Can you work these out from the model? Positions are in its coordinate system, mm. A direction names the side the tool comes from. Give positions to 0.01 mm unless a question says otherwise; leave off trailing zeros. Order: outer loops, then holes, each group sorted by start corner. A loop starts at its lowest first (then second) coordinate and runs counter-clockwise, first axis right, second up. Notation, with made-up numbers: M 21.25,68 L 58.25,68 A26 cw 58.25,98 Z; hole C 22.25,42.25 d7. An arc over 180 degrees is marked long. Answer as a JSON object with one key per item and string values.
```python
from build123d import *

# Parameters (mm, degrees)
F0_W     = 63.144043088
F0_H     = 24.9639227986
F1_DEPTH = 25.4
F2_W     = 1.27
F2_H     = 10.16
F3_DEPTH = 3.175
F4_W     = 10.16
F4_H     = 1.27
F5_DEPTH = 3.175


# Not quite as in the source:
# - a feature names something its author has since deleted; it is built from what else it names


with BuildPart() as f1:
    # F0 (on Front) → F1 (new body, symmetric)
    with BuildSketch(Plane.XZ):
        Rectangle(F0_W, F0_H)
    extrude(amount=F1_DEPTH, both=True)

    # F2 (on Front) → F3 (join, symmetric)
    with BuildSketch(Plane.XZ):
        with Locations((29.0800049829, 17.5400783525)):
            Rectangle(F2_W, F2_H)
    extrude(amount=F3_DEPTH, both=True)

    # F4 (on Front) → F5 (join, symmetric)
    with BuildSketch(Plane.XZ):
        with Locations((-36.6476550698, -9.8343824477)):
            Rectangle(F4_W, F4_H)
    extrude(amount=F5_DEPTH, both=True)


solid = f1.part
```
1) I want a section at A-A on y = -1. Write out the boundary of the cut face in (x, z) (3 decimals), and give its area (3 significant figures).
Results found:
{"outline": "M -41.728,-10.469 L -31.572,-10.469 L -31.572,-12.482 L 31.572,-12.482 L 31.572,12.482 L 29.715,12.482 L 29.715,22.62 L 28.445,22.62 L 28.445,12.482 L -31.572,12.482 L -31.572,-9.199 L -41.728,-9.199 Z", "area": "1,600 mm²"}
2) For faces 1 (the face through (-37, 0, -10.469)), 2 (the face through (29.715, 0, 17)), 3 (the face through (0, 0, -12.482)), 4 (the face through (-37, 0, -9.199)), which set-ups out of +Z, -Z, +X, -X, +Y, -Y let a thin tool reach every point of the face, with its end or its side?
Results found:
{"face 1": "-Z, -X, +Y, -Y", "face 2": "+Z, +X, +Y, -Y", "face 3": "-Z, +X, -X, +Y, -Y", "face 4": "+Z, -X, +Y, -Y"}
3) I'm going to push flat-ended pins straight in: pin 1 Ø1 at (x, z) = (-37.5, -10) entering from +Y (3 decimals); pin 2 Ø0.6 at (x, z) = (29, 16) entering from -Y (3 decimals); pin 3 Ø6 at (x, y) = (-29, -11) entering from +Z. Where does each tip first touch, or does it pass through?
Results found:
{"pin 1": "stops at y = 3.175", "pin 2": "stops at y = -3.175", "pin 3": "stops at z = 12.48"}
4) I need wall thicknesses on L1, parallel to Z at x = 19.5, y = 4.5; L2, parallel to X at y = 1.5, z = 11; L3, parallel to X at y = 0, z = 16 (3 decimals). Which ranges of each line are inside material? Lowest first, please.
Results found:
{"L1": "z = -12.48 to 12.48", "L2": "x = -31.57 to 31.57", "L3": "x = 28.445 to 29.715"}
5) I want a section at B-B on z = 20. Write out the boundary of the cut face in (x, y) (3 decimals), and give its area (3 significant figures).
Results found:
{"outline": "M 28.445,-3.175 L 29.715,-3.175 L 29.715,3.175 L 28.445,3.175 Z", "area": "8.06 mm²"}
6) I want a section at C-C on x = -33.5. Write out the boundary of the cut face in (y, z) (3 decimals), and give its area (3 significant figures).
Results found:
{"outline": "M -3.175,-10.469 L 3.175,-10.469 L 3.175,-9.199 L -3.175,-9.199 Z", "area": "8.06 mm²"}
